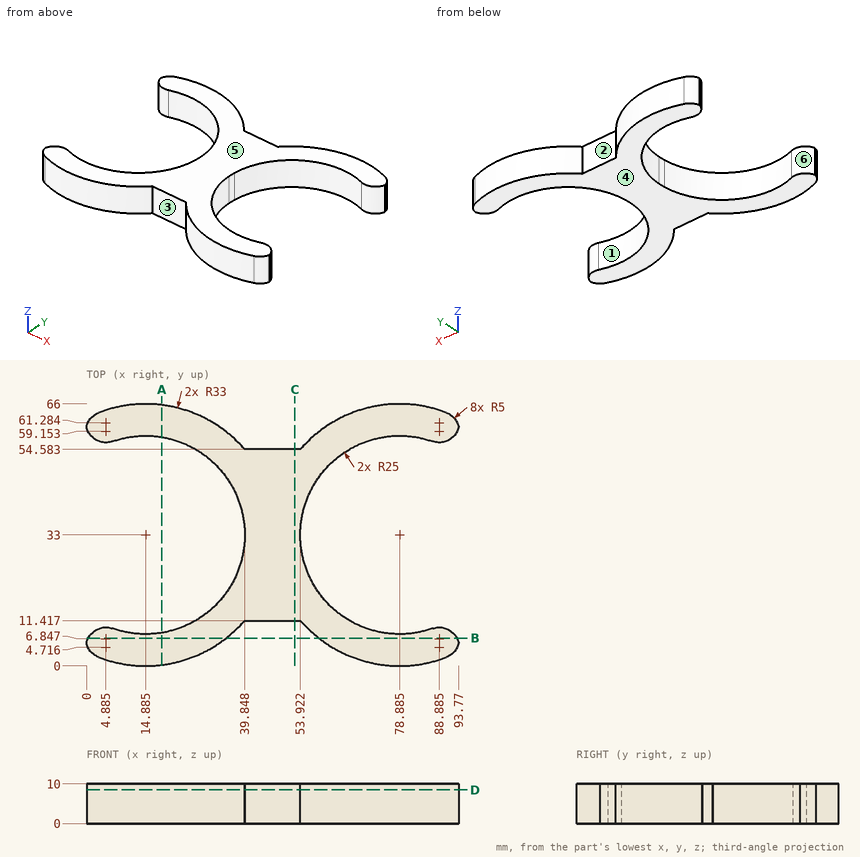
Source: three-view drawing plus pictorial views. Frame: mm from the lowest corner of the part. A direction names the side the tool comes from. Give positions to 0.01 mm unless a question says otherwise; leave off trailing zeros. Order: outer loops, then holes, each group sorted by start corner. A loop starts at its lowest first (then second) coordinate and runs counter-clockwise, first axis right, second up. Notation, with made-up numbers: (87.5, -33.75) - (105.5, -33.75) arc R31 cw to (105.5, -8.75) - close; hole circle Ø9 at (40, 63.5). An arc over 180 degrees is marked (long way). Put each result on its own line as item: value.
Item 1: Draft query along X for the marked faces 5 and 6. Return one class per face: +X half, -X half, draft (parallel to the pull), parting line (faces both ways), or undercut.
Found:
face 5: draft
face 6: undercut
Item 2: Ray query, L1, parallel to Y at x = 18, z = 4.5 (1 decimal); L2, parallel to Y at x = 13, z = 0.5; L3, parallel to X at y = 33, z = 3.25. Return the intervals inside material, ascending. Write a range as from..to.
Found:
L1: y = 0.1..8.2, 57.8..65.9
L2: y = 0.05..8.07, 57.93..65.95
L3: x = 39.85..53.92
Item 3: Section query A-A, the plane x = 19. Return loops of the section in (y, z), then the cut area to 3 significant figures.
Found:
outline: (0.26, 0) - (8.34, 0) - (8.34, 10) - (0.26, 10) - close; (57.66, 0) - (65.74, 0) - (65.74, 10) - (57.66, 10) - close
area: 162 mm^2
Item 4: Section query C-C, the plane x = 52.5. Return loops of the section in (y, z), then the cut area to 3 significant figures.
Found:
outline: (11.42, 0) - (54.58, 0) - (54.58, 10) - (11.42, 10) - close
area: 432 mm^2
Item 5: Section query B-B, the plane y = 7. Return loops of the section in (x, z).
Found:
outline: (0.44, 0) - (35.21, 0) - (35.21, 10) - (0.44, 10) - close; (58.56, 0) - (93.33, 0) - (93.33, 10) - (58.56, 10) - close
Item 6: Section query D-D, the plane z = 8.5. Return loops of the section in (x, y) (1 decimal), then the cut area to 3 significant figures.
Found:
outline: (0, 5.8) arc R5 ccw to (3.1, 2.2) arc R33 ccw to (39.8, 11.4) - (53.9, 11.4) arc R33 ccw to (90.7, 2.2) arc R5 ccw to (93.8, 5.8) arc R5 ccw to (87.2, 9.4) arc R25 cw to (53.9, 31.6) - (53.9, 34.4) arc R25 cw to (87.2, 56.6) arc R5 ccw to (93.8, 60.2) arc R5 ccw to (90.7, 63.8) arc R33 ccw to (53.9, 54.6) - (39.8, 54.6) arc R33 ccw to (3.1, 63.8) arc R5 ccw to (0, 60.2) arc R5 ccw to (6.6, 56.6) arc R25 cw to (39.8, 34.4) - (39.8, 31.6) arc R25 cw to (6.6, 9.4) arc R5 ccw to start
area: 2,030 mm^2
Item 7: Access query for the marked faces 1, 2, 3 and 4. Directions: +Z, -Z, +X, -X, +Y, -Y. A direction counts if a zero-diameter tool reaches every point of the face in a straight line with its end or side. Return the directions, or none.
Found:
face 1: +Z, -Z
face 2: +Z, -Z, +Y
face 3: +Z, -Z, -Y
face 4: -Z, +X, -X, +Y, -Y
Item 8: Contact query for flat-ended pins moving along their axis: pin 1 (6 mm diameter, centred on x = 73.5, z = 3, fed in from +Y); pin 2 (3 mm diameter, centred on x = 64, z = 7, fed in from -Y); pin 3 (3 mm diameter, centred on y = 7.5, z = 2, fed in from +X); pin 4 (10 mm diameter, centred on x = 33.5, y = 27, fed in from -Z). Output: stop coordinate, or through.
Found:
pin 1: stops at y = 65.91
pin 2: stops at y = 2.84
pin 3: stops at x = 93.72
pin 4: passes through
